Can you work these out from the model? Positions are in its coordinate system, mm. Face numbers are marked on the shaded views. A direction names the side the tool comes from. Give positions to 0.01 mm unless a question says otherwise; leave off trailing zeros. Write each loop counter-clockwise with the first axis right and the second up, starting at its lowest first coordinate (ties: lowest second). Pieces come first, ordered by that corner, then holes.
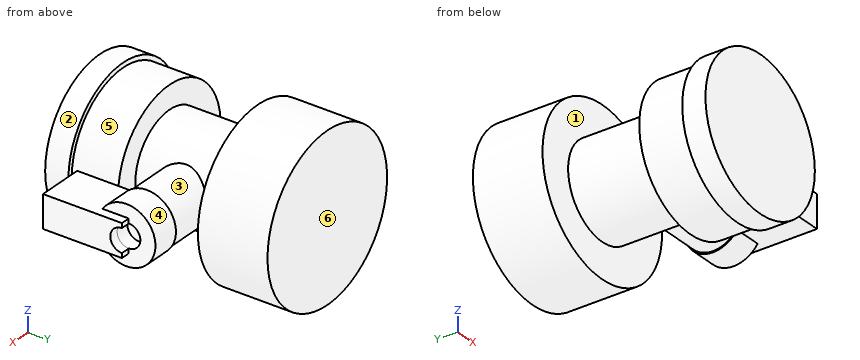
from build123d import *

# Parameters (mm, degrees)
SKETCH1_R                      = 10
BOSS_EXTRUDE1_DEPTH            = 19
SKETCH2_R                      = 6
BOSS_EXTRUDE2_DEPTH            = 19.5
SKETCH7_R                      = 15
BOSS_EXTRUDE9_DEPTH            = 10
SKETCH9_R                      = 16
BOSS_EXTRUDE10_DEPTH           = 5
SKETCH10_R                     = 17.5
BOSS_EXTRUDE11_DEPTH           = 15
SKETCH11_R                     = 6.25
BOSS_EXTRUDE12_DEPTH           = 6
SKETCH12_W                     = 10
SKETCH12_H                     = 7
BOSS_EXTRUDE13_DEPTH           = 10
BOSS_EXTRUDE13_DEPTH_BACK      = 7
SKETCH13_R                     = 2.5
CUT_EXTRUDE1_DEPTH             = 3
CUT_EXTRUDE1_DIRECTION_2_REACH = 4


with BuildPart() as part:
    # Sketch1 → Boss-Extrude1 (new body)
    with BuildSketch(Plane(origin=(0, 0, 0), x_dir=(1, 0, 0), z_dir=(0, 1, 0))):
        Circle(SKETCH1_R)
    extrude(amount=BOSS_EXTRUDE1_DEPTH)

    # Sketch2 → Boss-Extrude2 (add)
    with BuildSketch(Plane(origin=(0, 0, 0), x_dir=(0, 0, -1), z_dir=(1, 0, 0))):
        with Locations((0, 9.5)):
            Circle(SKETCH2_R)
    extrude(amount=BOSS_EXTRUDE2_DEPTH)

    # Sketch7 → Boss-Extrude9 (add)
    with BuildSketch(Plane.XZ):
        Circle(SKETCH7_R)
    extrude(amount=BOSS_EXTRUDE9_DEPTH)

    # Sketch9 → Boss-Extrude10 (add)
    with BuildSketch(Plane.XZ.offset(10)):
        Circle(SKETCH9_R)
    extrude(amount=BOSS_EXTRUDE10_DEPTH)

    # Sketch10 → Boss-Extrude11 (add)
    with BuildSketch(Plane(origin=(0, 19, 0), x_dir=(1, 0, 0), z_dir=(0, 1, 0))):
        Circle(SKETCH10_R)
    extrude(amount=BOSS_EXTRUDE11_DEPTH)

    # Sketch11 → Boss-Extrude12 (add)
    with BuildSketch(Plane(origin=(19.5, 0, 0), x_dir=(0, 0, -1), z_dir=(1, 0, 0))):
        with Locations((0, 9.5)):
            Circle(SKETCH11_R)
    extrude(amount=BOSS_EXTRUDE12_DEPTH)

    # Sketch12 → Boss-Extrude13 (add, two sides)
    with BuildSketch(Plane(origin=(0, 0, 0), x_dir=(1, 0, 0), z_dir=(0, 1, 0))) as boss_extrude13_sk:
        with Locations((22.5, 0)):
            Rectangle(SKETCH12_W, SKETCH12_H)
    extrude(amount=BOSS_EXTRUDE13_DEPTH)
    extrude(boss_extrude13_sk.sketch, amount=-BOSS_EXTRUDE13_DEPTH_BACK)

    # Sketch13 → Cut-Extrude1 (cut)
    with BuildSketch(Plane(origin=(25.5, 0, 0), x_dir=(0, 0, -1), z_dir=(1, 0, 0))):
        with Locations((0, 10)):
            Circle(SKETCH13_R)
    extrude(amount=-CUT_EXTRUDE1_DEPTH, mode=Mode.SUBTRACT)

    # Sketch13 → Cut-Extrude1 direction 2 (cut, up to next)
    with BuildSketch(Plane(origin=(25.5, 0, 0), x_dir=(0, 0, -1), z_dir=(1, 0, 0)), mode=Mode.PRIVATE) as cut_extrude1_direction_2_sk1:
        with Locations((0, 10)):
            Circle(SKETCH13_R)
    cut_extrude1_direction_2_tool1 = extrude(cut_extrude1_direction_2_sk1.sketch, amount=CUT_EXTRUDE1_DIRECTION_2_REACH, mode=Mode.PRIVATE) & part.part
    add(cut_extrude1_direction_2_tool1.solids().sort_by_distance((25.5, 10, 0))[0], mode=Mode.SUBTRACT)


solid = part.part
(1) If I drill on L1, parallel to Y at x = 8.5, z = -8.5; L2, parallel to Y at x = 23, z = 0; L3, parallel to Z at x = -0.5, y = 4, over which ranges is the centre line in solid material (lowest first)?
Returned:
L1: y = -15 to 0, 19 to 34
L2: y = -7 to 7.5, 12.5 to 15.75
L3: z = -9.99 to 9.99
(2) Imagine slicing it at A-A, the plane x = 23.5. Write out the boundary of the cut face in (y, z), plus the area to 3 significant figures.
Returned:
outline: (-7, -3.5) - (4.32, -3.5) arc R6.25 ccw (long way) to (4.32, 3.5) - (-7, 3.5) - close; hole circle Ø5 at (10, 0)
area: 177 mm2
(3) Imagine slicing it at C-C, the plane x = 0. Write out the boundary of the cut face in (y, z), plus the area to 4 significant figures.
Returned:
outline: (-15, -16) - (-10, -16) - (-10, -15) - (0, -15) - (0, -10) - (19, -10) - (19, -17.5) - (34, -17.5) - (34, 17.5) - (19, 17.5) - (19, 10) - (0, 10) - (0, 15) - (-10, 15) - (-10, 16) - (-15, 16) - close
area: 1,365 mm2
(4) Imagine slicing it at D-D, the plane z = 0. Write out the boundary of the cut face in (x, y), plus the area to 3 significant figures.
Returned:
outline: (-17.5, 19) - (-10, 19) - (-10, 0) - (-15, 0) - (-15, -10) - (-16, -10) - (-16, -15) - (16, -15) - (16, -10) - (15, -10) - (15, 0) - (10, 0) - (10, 3.5) - (17.5, 3.5) - (17.5, -7) - (27.5, -7) - (27.5, 7.5) - (22.5, 7.5) - (22.5, 12.5) - (25.5, 12.5) - (25.5, 15.75) - (19.5, 15.75) - (19.5, 15.5) - (10, 15.5) - (10, 19) - (17.5, 19) - (17.5, 34) - (-17.5, 34) - close
area: 1,650 mm2
(5) If we mould it in two halves opening along X, with no side actions, what happens to the marked faces 1, 2 and 3? For each: +X half, -X half, draft (parallel to the pull), parting line (faces both ways), or undercut.
Returned:
face 1: draft
face 2: parting line
face 3: undercut
(6) Will these pins go through, and if not, where does the flat tip stop? P1, Ø0.8, axis at x = 26, z = -3, coming from the +Y side; P2, Ø5.5, axis at y = 10, z = 1, coming from the +X side; P3, Ø7.5, axis at y = -4, z = 0, coming from the -X side; P4, Ø2, axis at y = 21, z = -1, coming from the +X side.
Returned:
P1: stops at y = 10
P2: stops at x = 27.5
P3: stops at x = -15
P4: stops at x = 17.5
(7) Imagine slicing it at B-B, the plane z = -14. Write out the boundary of the cut face in (x, y), plus the area to 3 significant figures.
Returned:
outline: (-10.5, 19) - (10.5, 19) - (10.5, 34) - (-10.5, 34) - close; (-7.75, -15) - (7.75, -15) - (7.75, -10) - (5.39, -10) - (5.39, 0) - (-5.39, 0) - (-5.39, -10) - (-7.75, -10) - close
area: 500 mm2
(8) For the marked faces 4, 5 and 6, which set-ups out of +Z, -Z, +X, -X, +Y, -Y let a thin tool reach every point of the face, with its end or its side?
Returned:
face 4: +X
face 5: none
face 6: +Z, -Z, +X, -X, +Y
